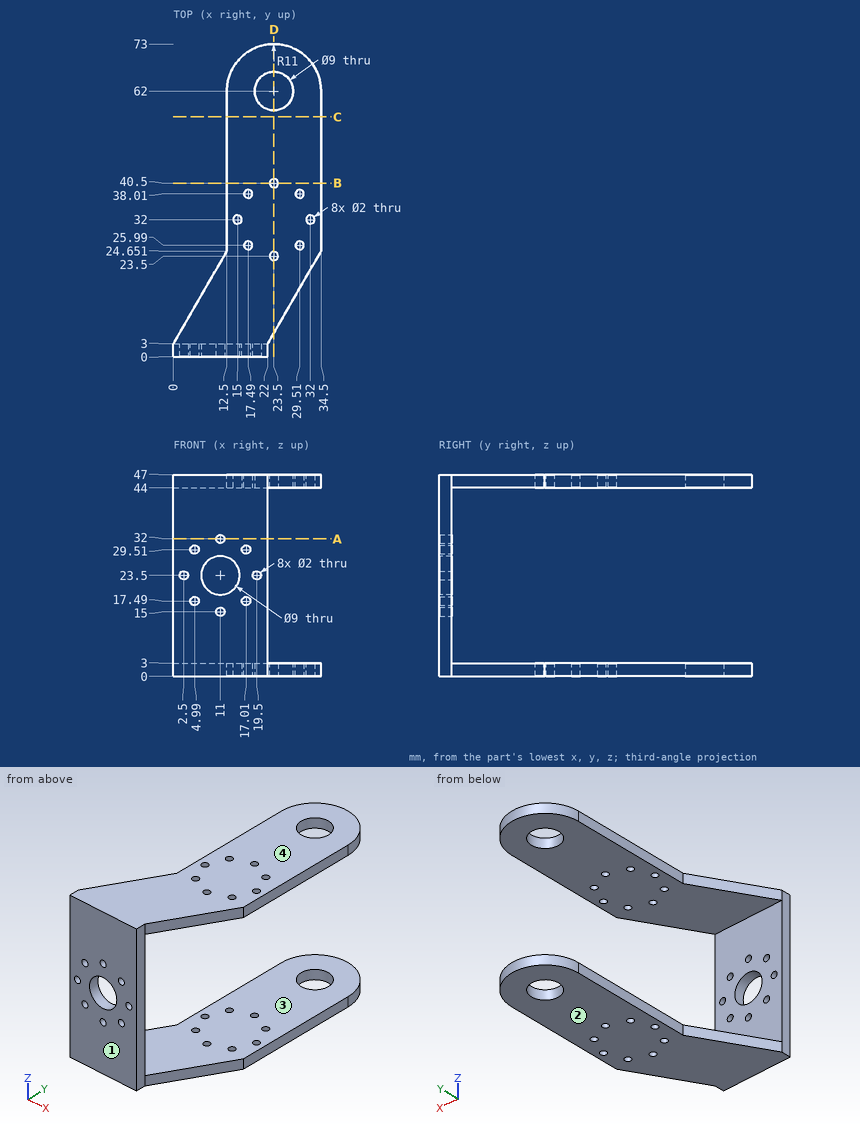
Source: three-view drawing plus pictorial views. Frame: mm from the lowest corner of the part. Give positions to 0.01 mm unless a question says otherwise; leave off trailing zeros. Order: outer loops, then holes, each group sorted by start corner. A loop starts at its lowest first (then second) coordinate and runs counter-clockwise, first axis right, second up. Notation, with made-up numbers: M 87.25,67.5 L 105.25,67.5 A18 ccw 105.25,94.5 Z; hole C 74,-22 d3. An arc over 180 degrees is marked long. Return JSON: item names as keys, results as strings.
1) Section query A-A on z = 32. Output: boundary loops of the cut face in (x, y).
Taken from the geometry:
{"outline": "M 0,0 L 10,0 L 10,3 L 0,3 Z; M 12,0 L 22,0 L 22,3 L 12,3 Z"}
2) Section query C-C on y = 56. Output: boundary loops of the cut face in (x, z), and give its area (3 significant figures).
Taken from the geometry:
{"outline": "M 12.5,0 L 34.5,0 L 34.5,3 L 12.5,3 Z; M 12.5,44 L 34.5,44 L 34.5,47 L 12.5,47 Z", "area": "132 mm2"}
3) Section query B-B on y = 40.5. Output: boundary loops of the cut face in (x, z).
Taken from the geometry:
{"outline": "M 12.5,0 L 22.5,0 L 22.5,3 L 12.5,3 Z; M 12.5,44 L 22.5,44 L 22.5,47 L 12.5,47 Z; M 24.5,0 L 34.5,0 L 34.5,3 L 24.5,3 Z; M 24.5,44 L 34.5,44 L 34.5,47 L 24.5,47 Z"}
4) Contact query for flat-ended pins moving along their axis: pin 1 (2.5 mm diameter, centred on x = 17.49, y = 38.01, fed in from +Z); pin 2 (1.5 mm diameter, centred on x = 15.5, z = 23, fed in from +Y); pin 3 (1.2 mm diameter, centred on x = 11, z = 15, fed in from +Y); pin 4 (3.5 mm diameter, centred on y = 48, z = 2, fed in from -X). Output: stop coordinate, or through.
Taken from the geometry:
{"pin 1": "stops at z = 47", "pin 2": "stops at y = 3", "pin 3": "passes through", "pin 4": "stops at x = 12.5"}
5) Mould query, pull axis Z, two halves, no side actions, for the marked faces 1, 2, 3 and 4. Classes: released by +Z, released by -Z, zero draft, split by the parting line, or undercut.
Taken from the geometry:
{"face 1": "zero draft", "face 2": "released by -Z", "face 3": "undercut", "face 4": "released by +Z"}
6) Section query D-D on x = 23.5. Count the separate pieces of the cut face and the enclosed holes in it.
Taken from the geometry:
{"separate pieces": "8", "enclosed holes": "0"}
7) Line query: L1, parallel to Z at x = 10, y = 9; L2, parallel to Y at x = 6.5, z = 33.5; L3, parallel to X at y = 62, z = 1.2. Output: solid intervals per line, ascending. Write a range as [from, to].
Taken from the geometry:
{"L1": "z = [0, 3], [44, 47]", "L2": "y = [0, 3]", "L3": "x = [12.5, 19], [28, 34.5]"}
